Build history of the part. All positions in model axes, mm. A direction names the side the tool comes from. Round coordinates to 2 decimals unless told otherwise and drop trailing zeros. Write each loop counter-clockwise with the first axis right and the second up, starting at its lowest first coordinate (ties: lowest second). Pieces come first, ordered by that corner, then holes. Notation, with made-up numbers: M 19.25,79 L 43.25,79 A30 ccw 43.25,109 Z; hole C -1,26.25 d5. An arc over 180 degrees is marked long. Write item = value, one per line. Start each with the question number.
Q1. Drop flat-ended pins along their axis: P1, Ø2, axis at y = 23.5, z = 9.5, coming from the -X side; P2, Ø8, axis at y = 25, z = -2, coming from the +X side; P3, Ø10, axis at x = -11, y = 10, coming from the +Z side. Give the stop position or say it passes through.
Q2. Band-saw the part on D-D on z = -20. Write the cut outline in (x, y), plus the area to 3 significant figures.
Q3. Band-saw the part on B-B on x = 0. Write the cut outline in (y, z), plus the area to 3 significant figures.
Q4. Probe L1, parallel to Y at x = -9.5, z = -24.5; L2, parallel to X at y = 16, z = 1.5; L3, parallel to X at y = 8, z = 0.5. List the from-to ranges inside material, lowest first.
Q5. Band-saw the part on C-C on y = 18. Write the cut outline in (x, z), plus the area to 3 significant figures.
Q6. Band-saw the part on A-A on z = 0. Write the cut outline in (x, y), plus the area to 3 significant figures.
Q7. Tool access for faces 1 (the flat face through (-1, -6, -28.293)), 2 (the cylindrical face through (3.755, 14.79, 11.923)): list every direction of +Z, -Z, +X, -X, +Y, -Y with a clear straight run to the whole face (end or side of a thin tool).
```python
from build123d import *

# Parameters (mm, degrees)
SKETCH_1_R      = 12.5
EXTRUDE_1_DEPTH = 30
SKETCH_2_W      = 42.461745146
SKETCH_2_H      = 56.586214178
EXTRUDE_2_DEPTH = 12


with BuildPart() as part:
    # Эскиз1 → Вытянуть1 (new body)
    with BuildSketch(Plane(origin=(0, 0, 0), x_dir=(1, 0, 0), z_dir=(0, 1, 0))):
        with Locations(Location((0, 0, 0), (0, 0, 270))):
            Circle(SKETCH_1_R)
    extrude(amount=EXTRUDE_1_DEPTH)

    # Эскиз2 → Вытянуть2 (add)
    with BuildSketch(Plane.XZ):
        with Locations((-0.627472581, 0)):
            Rectangle(SKETCH_2_W, SKETCH_2_H)
    extrude(amount=EXTRUDE_2_DEPTH)


solid = part.part
```
Conclusion:
q1.P1 = -9.17
q1.P2 = 12.5
q1.P3 = 10.97
q2.outline = M -21.86,-12 L 20.6,-12 L 20.6,0 L -21.86,0 Z
q2.area = 510 mm^2
q3.outline = M -12,-28.29 L 0,-28.29 L 0,-12.5 L 30,-12.5 L 30,12.5 L 0,12.5 L 0,28.29 L -12,28.29 Z
q3.area = 1,430 mm^2
q4.L1 = -12 to 0
q4.L2 = -12.41 to 12.41
q4.L3 = -12.49 to 12.49
q5.outline = C 0,0 d25
q5.area = 491 mm^2
q6.outline = M -21.86,-12 L 20.6,-12 L 20.6,0 L 12.5,0 L 12.5,30 L -12.5,30 L -12.5,0 L -21.86,0 Z
q6.area = 1,260 mm^2
q7.face_1 = -Z, +X, -X, +Y, -Y
q7.face_2 = +Y
